Geometry check sheet. Reference: the model listing, model coordinates, mm. Face numbers are marked on the shaded views. Coordinates: 2 decimals unless noted, no trailing zeros. Order: outer loops, then holes, each group sorted by start corner. A loop starts at its lowest first (then second) coordinate and runs counter-clockwise, first axis right, second up. Notation, with made-up numbers: (56, 5.5) - (111, 5.5) arc R16 ccw to (111, 31.5) - close; hole circle Ø6 at (45, 70.5). An arc over 180 degrees is marked (long way). Put each result on its own line as item: value.
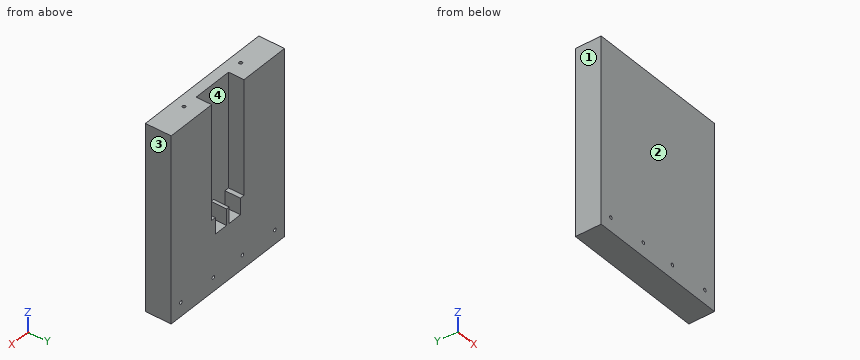
from build123d import *

# Parameters (mm, degrees)
BOSS_EXTRUDE2_DEPTH = 16.002
SKETCH1_6_W         = 25.4
SKETCH1_6_H         = 71.12
BOSS_EXTRUDE3_DEPTH = 6.35
SKETCH1_7_W         = 8.89
SKETCH1_7_H         = 10.16
BOSS_EXTRUDE4_DEPTH = 6.35
SKETCH4_R           = 1.016
CUT_EXTRUDE2_DEPTH  = 17.002
SKETCH5_R           = 1.016
CUT_EXTRUDE3_DEPTH  = 12.7


with BuildPart() as part:
    # Sketch1 → Boss-Extrude2 (new body)
    with BuildSketch(Plane(origin=(0, 0, 0), x_dir=(1, 0, 0), z_dir=(0, 1, 0))):
        Polygon((0, 115.57), (0, 0), (31.75, 0), (31.75, 71.12), (34.56, 71.12), (34.56, 81.28), (43.45, 81.28), (43.45, 71.12), (45.45, 71.12), (45.45, 81.28), (54.34, 81.28), (54.34, 71.12), (57.15, 71.12), (57.15, 0), (88.9, 0), (88.9, 115.57), align=None)
    extrude(amount=BOSS_EXTRUDE2_DEPTH)



with BuildPart() as body_2:
    # Sketch1_6 → Boss-Extrude3 (new body)
    with BuildSketch(Plane(origin=(0, 0, 0), x_dir=(1, 0, 0), z_dir=(0, 1, 0))):
        with Locations((44.45, 35.56)):
            Rectangle(SKETCH1_6_W, SKETCH1_6_H)
    extrude(amount=BOSS_EXTRUDE3_DEPTH)


with BuildPart() as part_1:
    add(part.part)

    add(body_2.part)  # Boss-Extrude4 merges body 2
    # Sketch1_7 → Boss-Extrude4 (add)
    with BuildSketch(Plane(origin=(0, 0, 0), x_dir=(1, 0, 0), z_dir=(0, 1, 0))):
        with Locations((39.005, 76.2)):
            Rectangle(SKETCH1_7_W, SKETCH1_7_H)
        with Locations((49.895, 76.2)):
            Rectangle(SKETCH1_7_W, SKETCH1_7_H)
    extrude(amount=BOSS_EXTRUDE4_DEPTH)

    # Sketch4 → Cut-Extrude2 (cut, through all)
    with BuildSketch(Plane(origin=(0, 16.002, 0), x_dir=(1, 0, 0), z_dir=(0, 1, 0))):
        with Locations((7.62, 106.934)):
            Circle(SKETCH4_R)
        with Locations((33.02, 106.934)):
            Circle(SKETCH4_R)
        with Locations((55.88, 106.934)):
            Circle(SKETCH4_R)
        with Locations((81.28, 106.934)):
            Circle(SKETCH4_R)
    extrude(amount=-CUT_EXTRUDE2_DEPTH, mode=Mode.SUBTRACT)

    # Sketch5 → Cut-Extrude3 (cut)
    with BuildSketch(Plane.XY):
        with Locations((22.225, 6.35)):
            Circle(SKETCH5_R)
        with Locations((66.675, 6.35)):
            Circle(SKETCH5_R)
    extrude(amount=-CUT_EXTRUDE3_DEPTH, mode=Mode.SUBTRACT)


solid = part_1.part
Q1. Draft check along X on the marked faces 1, 2, 3 and 4. Enter one of: pulls with the +X half, pulls with the -X half, needs draft (parallel to the pull), parting line crosses it, or undercut.
Answer block:
face 1: pulls with the -X half
face 2: needs draft
face 3: pulls with the +X half
face 4: undercut
Q2. Section check B-B on y = 12.75. Record the boundary of the cut face in (x, z), then the cut area to 3 significant figures.
Answer block:
outline: (0, -115.57) - (88.9, -115.57) - (88.9, 0) - (57.15, 0) - (57.15, -71.12) - (54.34, -71.12) - (54.34, -81.28) - (45.45, -81.28) - (45.45, -71.12) - (43.45, -71.12) - (43.45, -81.28) - (34.56, -81.28) - (34.56, -71.12) - (31.75, -71.12) - (31.75, 0) - (0, 0) - close; hole circle Ø2.03 at (7.62, -106.93); hole circle Ø2.03 at (33.02, -106.93); hole circle Ø2.03 at (55.88, -106.93); hole circle Ø2.03 at (81.28, -106.93)
area: 8,270 mm^2
Q3. Thickness scan on L1, parallel to X at y = 5.25, z = -107; L2, parallel to Z at x = 33.02, y = 6.5; L3, parallel to Z at x = 7.62, y = 8.75. Record the ranges inside material, lowest first. Write a range as [from, to].
Answer block:
L1: x = [0, 6.61], [8.63, 32.01], [34.03, 54.87], [56.89, 80.27], [82.29, 88.9]
L2: z = [-115.57, -107.95], [-105.92, -71.12]
L3: z = [-115.57, -107.95], [-105.92, 0]
Q4. Depth check by flat-ended pin: pin 1 Ø4.5 at (x, y) = (38, 12) entering from +Z; pin 2 Ø12.5 at (x, z) = (41, -28.5) entering from +Y; pin 3 Ø1.2 at (x, z) = (81.28, -106.934) entering from +Y; pin 4 Ø1.6 at (x, y) = (44.5, 9.5) entering from +Z. Enter the tip coordinate at first touch or a pass-through.
Answer block:
pin 1: stops at z = -81.28
pin 2: stops at y = 6.35
pin 3: passes through
pin 4: stops at z = -71.12
Q5. Section check A-A on z = -18. Record the boundary of the cut face in (x, y).
Answer block:
outline: (0, 0) - (88.9, 0) - (88.9, 16) - (57.15, 16) - (57.15, 6.35) - (31.75, 6.35) - (31.75, 16) - (0, 16) - close
